from build123d import *

# Parameters (mm, degrees)
SKETCH1_W               = 180
SKETCH1_H               = 80
BOSS_EXTRUDE1_DEPTH     = 3
CUT_EXTRUDE_THIN1_DEPTH = 5


with BuildPart() as part:
    # Sketch1 → Boss-Extrude1 (new body)
    with BuildSketch(Plane(origin=(0, 0, 0), x_dir=(1, 0, 0), z_dir=(0, 1, 0))):
        with Locations((90, 40)):
            Rectangle(SKETCH1_W, SKETCH1_H)
    extrude(amount=BOSS_EXTRUDE1_DEPTH)

    # Sketch1<3> → Cut-Extrude-Thin1 (cut, symmetric)
    with BuildSketch(Plane(origin=(0, 0, 0), x_dir=(1, 0, 0), z_dir=(0, 1, 0))):
        with BuildLine():
            ThreePointArc((136.5, 66.174335789), (134, 63.674335789), (131.5, 66.174335789))
            ThreePointArc((131.5, 66.174335789), (126, 71.674335789), (120.5, 66.174335789))
            ThreePointArc((120.5, 66.174335789), (118, 63.674335789), (115.5, 66.174335789))
            ThreePointArc((115.5, 66.174335789), (110, 71.674335789), (104.5, 66.174335789))
            ThreePointArc((104.5, 66.174335789), (102, 63.674335789), (99.5, 66.174335789))
            ThreePointArc((99.5, 66.174335789), (94, 71.674335789), (88.5, 66.174335789))
            ThreePointArc((88.5, 66.174335789), (86, 63.674335789), (83.5, 66.174335789))
            ThreePointArc((83.5, 66.174335789), (78, 71.674335789), (72.5, 66.174335789))
            ThreePointArc((72.5, 66.174335789), (70, 63.674335789), (67.5, 66.174335789))
            ThreePointArc((67.5, 66.174335789), (62, 71.674335789), (56.5, 66.174335789))
            ThreePointArc((56.5, 66.174335789), (54, 63.674335789), (51.5, 66.174335789))
            ThreePointArc((51.5, 66.174335789), (46, 71.674335789), (40.5, 66.174335789))
            Line((40.5, 66.174335789), (43.5, 66.174335789))
            ThreePointArc((43.5, 66.174335789), (46, 68.674335789), (48.5, 66.174335789))
            ThreePointArc((48.5, 66.174335789), (54, 60.674335789), (59.5, 66.174335789))
            ThreePointArc((59.5, 66.174335789), (62, 68.674335789), (64.5, 66.174335789))
            ThreePointArc((64.5, 66.174335789), (70, 60.674335789), (75.5, 66.174335789))
            ThreePointArc((75.5, 66.174335789), (78, 68.674335789), (80.5, 66.174335789))
            ThreePointArc((80.5, 66.174335789), (86, 60.674335789), (91.5, 66.174335789))
            ThreePointArc((91.5, 66.174335789), (94, 68.674335789), (96.5, 66.174335789))
            ThreePointArc((96.5, 66.174335789), (102, 60.674335789), (107.5, 66.174335789))
            ThreePointArc((107.5, 66.174335789), (110, 68.674335789), (112.5, 66.174335789))
            ThreePointArc((112.5, 66.174335789), (118, 60.674335789), (123.5, 66.174335789))
            ThreePointArc((123.5, 66.174335789), (126, 68.674335789), (128.5, 66.174335789))
            ThreePointArc((128.5, 66.174335789), (134, 60.674335789), (139.5, 66.174335789))
            Line((139.5, 66.174335789), (136.5, 66.174335789))
        make_face()
        with BuildLine():
            ThreePointArc((136.5, 50.174335789), (134, 47.674335789), (131.5, 50.174335789))
            ThreePointArc((131.5, 50.174335789), (126, 55.674335789), (120.5, 50.174335789))
            ThreePointArc((120.5, 50.174335789), (118, 47.674335789), (115.5, 50.174335789))
            ThreePointArc((115.5, 50.174335789), (110, 55.674335789), (104.5, 50.174335789))
            ThreePointArc((104.5, 50.174335789), (102, 47.674335789), (99.5, 50.174335789))
            ThreePointArc((99.5, 50.174335789), (94, 55.674335789), (88.5, 50.174335789))
            ThreePointArc((88.5, 50.174335789), (86, 47.674335789), (83.5, 50.174335789))
            ThreePointArc((83.5, 50.174335789), (78, 55.674335789), (72.5, 50.174335789))
            ThreePointArc((72.5, 50.174335789), (70, 47.674335789), (67.5, 50.174335789))
            ThreePointArc((67.5, 50.174335789), (62, 55.674335789), (56.5, 50.174335789))
            ThreePointArc((56.5, 50.174335789), (54, 47.674335789), (51.5, 50.174335789))
            ThreePointArc((51.5, 50.174335789), (46, 55.674335789), (40.5, 50.174335789))
            Line((40.5, 50.174335789), (43.5, 50.174335789))
            ThreePointArc((43.5, 50.174335789), (46, 52.674335789), (48.5, 50.174335789))
            ThreePointArc((48.5, 50.174335789), (54, 44.674335789), (59.5, 50.174335789))
            ThreePointArc((59.5, 50.174335789), (62, 52.674335789), (64.5, 50.174335789))
            ThreePointArc((64.5, 50.174335789), (70, 44.674335789), (75.5, 50.174335789))
            ThreePointArc((75.5, 50.174335789), (78, 52.674335789), (80.5, 50.174335789))
            ThreePointArc((80.5, 50.174335789), (86, 44.674335789), (91.5, 50.174335789))
            ThreePointArc((91.5, 50.174335789), (94, 52.674335789), (96.5, 50.174335789))
            ThreePointArc((96.5, 50.174335789), (102, 44.674335789), (107.5, 50.174335789))
            ThreePointArc((107.5, 50.174335789), (110, 52.674335789), (112.5, 50.174335789))
            ThreePointArc((112.5, 50.174335789), (118, 44.674335789), (123.5, 50.174335789))
            ThreePointArc((123.5, 50.174335789), (126, 52.674335789), (128.5, 50.174335789))
            ThreePointArc((128.5, 50.174335789), (134, 44.674335789), (139.5, 50.174335789))
            Line((139.5, 50.174335789), (136.5, 50.174335789))
        make_face()
        with BuildLine():
            ThreePointArc((136.5, 34.174335789), (134, 31.674335789), (131.5, 34.174335789))
            ThreePointArc((131.5, 34.174335789), (126, 39.674335789), (120.5, 34.174335789))
            ThreePointArc((120.5, 34.174335789), (118, 31.674335789), (115.5, 34.174335789))
            ThreePointArc((115.5, 34.174335789), (110, 39.674335789), (104.5, 34.174335789))
            ThreePointArc((104.5, 34.174335789), (102, 31.674335789), (99.5, 34.174335789))
            ThreePointArc((99.5, 34.174335789), (94, 39.674335789), (88.5, 34.174335789))
            ThreePointArc((88.5, 34.174335789), (86, 31.674335789), (83.5, 34.174335789))
            ThreePointArc((83.5, 34.174335789), (78, 39.674335789), (72.5, 34.174335789))
            ThreePointArc((72.5, 34.174335789), (70, 31.674335789), (67.5, 34.174335789))
            ThreePointArc((67.5, 34.174335789), (62, 39.674335789), (56.5, 34.174335789))
            ThreePointArc((56.5, 34.174335789), (54, 31.674335789), (51.5, 34.174335789))
            ThreePointArc((51.5, 34.174335789), (46, 39.674335789), (40.5, 34.174335789))
            Line((40.5, 34.174335789), (43.5, 34.174335789))
            ThreePointArc((43.5, 34.174335789), (46, 36.674335789), (48.5, 34.174335789))
            ThreePointArc((48.5, 34.174335789), (54, 28.674335789), (59.5, 34.174335789))
            ThreePointArc((59.5, 34.174335789), (62, 36.674335789), (64.5, 34.174335789))
            ThreePointArc((64.5, 34.174335789), (70, 28.674335789), (75.5, 34.174335789))
            ThreePointArc((75.5, 34.174335789), (78, 36.674335789), (80.5, 34.174335789))
            ThreePointArc((80.5, 34.174335789), (86, 28.674335789), (91.5, 34.174335789))
            ThreePointArc((91.5, 34.174335789), (94, 36.674335789), (96.5, 34.174335789))
            ThreePointArc((96.5, 34.174335789), (102, 28.674335789), (107.5, 34.174335789))
            ThreePointArc((107.5, 34.174335789), (110, 36.674335789), (112.5, 34.174335789))
            ThreePointArc((112.5, 34.174335789), (118, 28.674335789), (123.5, 34.174335789))
            ThreePointArc((123.5, 34.174335789), (126, 36.674335789), (128.5, 34.174335789))
            ThreePointArc((128.5, 34.174335789), (134, 28.674335789), (139.5, 34.174335789))
            Line((139.5, 34.174335789), (136.5, 34.174335789))
        make_face()
        with BuildLine():
            ThreePointArc((136.5, 18.174335789), (134, 15.674335789), (131.5, 18.174335789))
            ThreePointArc((131.5, 18.174335789), (126, 23.674335789), (120.5, 18.174335789))
            ThreePointArc((120.5, 18.174335789), (118, 15.674335789), (115.5, 18.174335789))
            ThreePointArc((115.5, 18.174335789), (110, 23.674335789), (104.5, 18.174335789))
            ThreePointArc((104.5, 18.174335789), (102, 15.674335789), (99.5, 18.174335789))
            ThreePointArc((99.5, 18.174335789), (94, 23.674335789), (88.5, 18.174335789))
            ThreePointArc((88.5, 18.174335789), (86, 15.674335789), (83.5, 18.174335789))
            ThreePointArc((83.5, 18.174335789), (78, 23.674335789), (72.5, 18.174335789))
            ThreePointArc((72.5, 18.174335789), (70, 15.674335789), (67.5, 18.174335789))
            ThreePointArc((67.5, 18.174335789), (62, 23.674335789), (56.5, 18.174335789))
            ThreePointArc((56.5, 18.174335789), (54, 15.674335789), (51.5, 18.174335789))
            ThreePointArc((51.5, 18.174335789), (46, 23.674335789), (40.5, 18.174335789))
            Line((40.5, 18.174335789), (43.5, 18.174335789))
            ThreePointArc((43.5, 18.174335789), (46, 20.674335789), (48.5, 18.174335789))
            ThreePointArc((48.5, 18.174335789), (54, 12.674335789), (59.5, 18.174335789))
            ThreePointArc((59.5, 18.174335789), (62, 20.674335789), (64.5, 18.174335789))
            ThreePointArc((64.5, 18.174335789), (70, 12.674335789), (75.5, 18.174335789))
            ThreePointArc((75.5, 18.174335789), (78, 20.674335789), (80.5, 18.174335789))
            ThreePointArc((80.5, 18.174335789), (86, 12.674335789), (91.5, 18.174335789))
            ThreePointArc((91.5, 18.174335789), (94, 20.674335789), (96.5, 18.174335789))
            ThreePointArc((96.5, 18.174335789), (102, 12.674335789), (107.5, 18.174335789))
            ThreePointArc((107.5, 18.174335789), (110, 20.674335789), (112.5, 18.174335789))
            ThreePointArc((112.5, 18.174335789), (118, 12.674335789), (123.5, 18.174335789))
            ThreePointArc((123.5, 18.174335789), (126, 20.674335789), (128.5, 18.174335789))
            ThreePointArc((128.5, 18.174335789), (134, 12.674335789), (139.5, 18.174335789))
            Line((139.5, 18.174335789), (136.5, 18.174335789))
        make_face()
    extrude(amount=CUT_EXTRUDE_THIN1_DEPTH, both=True, mode=Mode.SUBTRACT)


solid = part.part
Design review of the part built by this model. Coordinates are the model's own, in mm. Give positions to 0.01 mm unless a question says otherwise; leave off trailing zeros. Order: outer loops, then holes, each group sorted by start corner. A loop starts at its lowest first (then second) coordinate and runs counter-clockwise, first axis right, second up.
1. Add section A-A, the plane x = 126. State the section outline as (y, z) points.
Solution:
outline: (0, -80) - (3, -80) - (3, -71.67) - (0, -71.67) - close; (0, -68.67) - (3, -68.67) - (3, -55.67) - (0, -55.67) - close; (0, -52.67) - (3, -52.67) - (3, -39.67) - (0, -39.67) - close; (0, -36.67) - (3, -36.67) - (3, -23.67) - (0, -23.67) - close; (0, -20.67) - (3, -20.67) - (3, 0) - (0, 0) - close
2. Add section B-B, the plane y = 2.4. State how many separate pieces and enclosed holes the cut face has, then the cut area to 3 significant figures.
Solution:
separate pieces: 1
enclosed holes: 4
area: 12,600 mm2
3. Add section C-C, the plane x = 85.5. State the section outline as (y, z) points.
Solution:
outline: (0, -80) - (3, -80) - (3, -63.72) - (0, -63.72) - close; (0, -60.7) - (3, -60.7) - (3, -47.72) - (0, -47.72) - close; (0, -44.7) - (3, -44.7) - (3, -31.72) - (0, -31.72) - close; (0, -28.7) - (3, -28.7) - (3, -15.72) - (0, -15.72) - close; (0, -12.7) - (3, -12.7) - (3, 0) - (0, 0) - close
4. To check wall thickness, follow L1, parallel to Z at x = 116, y = 2; L2, parallel to Z at x = 69, y = 0.35. State the ranges of each line that lie inside material, in increasing order.
Solution:
L1: z = -80 to -64.67, -61.05 to -48.67, -45.05 to -32.67, -29.05 to -16.67, -13.05 to 0
L2: z = -80 to -63.88, -60.77 to -47.88, -44.77 to -31.88, -28.77 to -15.88, -12.77 to 0
5. For pin 1 Ø1.5 at (x, z) = (64, -53) entering from +Y, flat-tipped, find the tip position at first contact; note if it passes through.
Solution:
pin 1: passes through
6. Mouldability with a two-part tool opening along Z and no side actions: class faces 1 (the cylindrical face through (125.945, 1.479, -68.674)), 2 (the cylindrical face through (69.879, 1.479, -28.676)) as +Z half, -Z half, draft (parallel to the pull), parting line (faces both ways), or undercut.
Solution:
face 1: undercut
face 2: undercut
